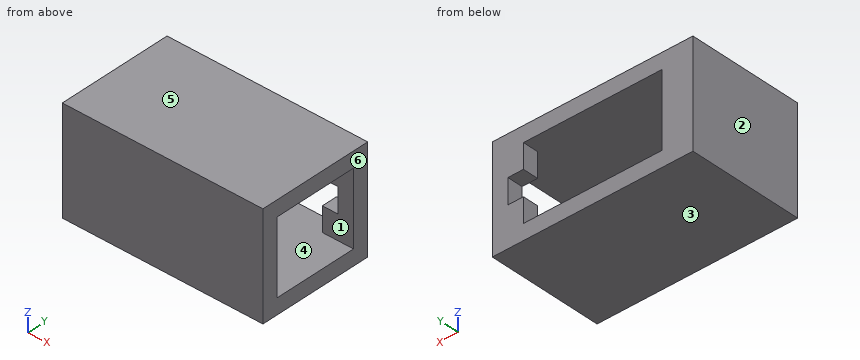
```python
from build123d import *

# Parameters (mm, degrees)
SKETCH2_W           = 32.2
SKETCH2_H           = 16.8
BOSS_EXTRUDE1_DEPTH = 18.5
SKETCH3_W           = 22.2
SKETCH3_H           = 11.8
CUT_EXTRUDE1_DEPTH  = 16
SKETCH4_W           = 11.8
SKETCH4_H           = 13.5
CUT_EXTRUDE2_DEPTH  = 5
SKETCH5_W           = 2.5
SKETCH5_H           = 4
CUT_EXTRUDE3_DEPTH  = 2.5


with BuildPart() as part:
    # Sketch2 → Boss-Extrude1 (new body)
    with BuildSketch(Plane(origin=(0, 0, 0), x_dir=(1, 0, 0), z_dir=(0, 1, 0))):
        Rectangle(SKETCH2_W, SKETCH2_H)
    extrude(amount=-BOSS_EXTRUDE1_DEPTH)

    # Sketch3 → Cut-Extrude1 (cut)
    with BuildSketch(Plane(origin=(0, 0, 0), x_dir=(1, 0, 0), z_dir=(0, 1, 0))):
        Rectangle(SKETCH3_W, SKETCH3_H)
    extrude(amount=-CUT_EXTRUDE1_DEPTH, mode=Mode.SUBTRACT)

    # Sketch4 → Cut-Extrude2 (cut)
    with BuildSketch(Plane(origin=(16.1, 0, 0), x_dir=(0, 0, -1), z_dir=(1, 0, 0))):
        with Locations((0, -9.25)):
            Rectangle(SKETCH4_W, SKETCH4_H)
    extrude(amount=-CUT_EXTRUDE2_DEPTH, mode=Mode.SUBTRACT)

    # Sketch5 → Cut-Extrude3 (cut)
    with BuildSketch(Plane(origin=(0, 0, 0), x_dir=(1, 0, 0), z_dir=(0, 1, 0))):
        with Locations((12.35, 0)):
            Rectangle(SKETCH5_W, SKETCH5_H)
    extrude(amount=-CUT_EXTRUDE3_DEPTH, mode=Mode.SUBTRACT)


solid = part.part
```
Work out the finished part from the listing and answer in its coordinate system (mm). Face numbers are marked on the shaded views. A direction names the side the tool comes from. Give positions to 0.01 mm unless a question says otherwise; leave off trailing zeros. Loops run counter-clockwise (first coordinate to the right, second up) from the corner with the lowest first, then second, coordinate; pieces in that order, holes last. Notation, with made-up numbers: (22.25, 10) - (39.25, 10) arc R29 cw to (39.25, 30) - close; hole circle Ø8 at (-35, 74). An arc over 180 degrees is marked (long way). One line per question, with ' | ' between items.
(1) The part is cut by section A-A (z = 1.5). Write down the section's boundary in (x, y).
Recorded:
outline: (-16.1, -18.5) - (16.1, -18.5) - (16.1, -16) - (-11.1, -16) - (-11.1, 0) - (-16.1, 0) - close; (13.6, -2.5) - (16.1, -2.5) - (16.1, 0) - (13.6, 0) - close
(2) The mould has two halves that part along Z. Classify the marked faces 3, 4, 5 and 6: +Z half, -Z half, draft (parallel to the pull), parting line (faces both ways), or undercut.
Recorded:
face 3: -Z half | face 4: undercut | face 5: +Z half | face 6: draft
(3) A tool of negligible diameter and unlimited length cuts with its end or side. For the marked faces 1 and 2, from which of +Z, -Z, +X, -X, +Y, -Y can it reach the whole face along a straight path? Write none if from no direction.
Recorded:
face 1: +X | face 2: +Z, -Z, -X, +Y, -Y
(4) Straight lines are drawn through the part: probe 1 along Z at (x, y) = (6.5, -11.5); probe 2 along X at (y, z) = (-1, 4); probe 3 along Y at (x, z) = (13, 4.75). For each, find the intervals that lie inside material, in ascending order.
Recorded:
probe 1: z = -8.4 to -5.9, 5.9 to 8.4 | probe 2: x = -16.1 to -11.1, 11.1 to 16.1 | probe 3: y = -18.5 to -16, -2.5 to 0
(5) The part is cut by section B-B (x = 14). Write down the section's boundary in (y, z), then the cut area to 4 significant figures.
Recorded:
outline: (-18.5, -8.4) - (0, -8.4) - (0, 8.4) - (-18.5, 8.4) - close; hole (-16, -5.9) - (-2.5, -5.9) - (-2.5, 5.9) - (-16, 5.9) - close | area: 151.5 mm²
(6) Each of these flat-tipped pins is pushed along its axis until it touches: pin 1 Ø3.5 at (x, z) = (7.5, -0.5) entering from +Y; pin 2 Ø9.5 at (y, z) = (-11, -1) entering from +X. Where does it stop, or does it pass through?
Recorded:
pin 1: stops at y = -16 | pin 2: stops at x = -11.1
(7) The part is cut by section C-C (y = -6). Write down the section's boundary in (x, z), then the cut area to 3 significant figures.
Recorded:
outline: (-16.1, -8.4) - (16.1, -8.4) - (16.1, -5.9) - (-11.1, -5.9) - (-11.1, 5.9) - (16.1, 5.9) - (16.1, 8.4) - (-16.1, 8.4) - close | area: 220 mm²
(8) The part is cut by section D-D (x = -1.5). Write down the section's boundary in (y, z), then the cut area to 3 significant figures.
Recorded:
outline: (-18.5, -8.4) - (0, -8.4) - (0, -5.9) - (-16, -5.9) - (-16, 5.9) - (0, 5.9) - (0, 8.4) - (-18.5, 8.4) - close | area: 122 mm²
